```python
from build123d import *

# Parameters (mm, degrees)
F0_W     = 304.8
F0_H     = 381
F1_DEPTH = 482.6
F2_R     = 25.4
F3_R     = 12.7
F4_DEPTH = 25.4


# Not quite as in the source:
# - the program builds the solid bodies; features that only make, move or delete a surface that nothing else refers to are left out


with BuildPart() as f1:
    # F0 (on Top) → F1 (new body)
    with BuildSketch(Plane.XY):
        Rectangle(F0_W, F0_H)
    extrude(amount=F1_DEPTH)

    # F2
    f2_edges = [f1.edges().sort_by_distance(p)[0] for p in [
        (-152.4, 0, 482.6),
        (152.4, 0, 482.6),
    ]]
    fillet(f2_edges, radius=F2_R)

    # F3
    f3_edges = [f1.edges().sort_by_distance(p)[0] for p in [
        (-152.4, -190.5, 228.6),
        (-144.960512, -190.5, 475.160512),
        (0, -190.5, 482.6),
        (144.960512, -190.5, 475.160512),
        (152.4, -190.5, 228.6),
    ]]
    fillet(f3_edges, radius=F3_R)

    # F4 (cut): a face of the model
    f4_faces = [f1.faces().sort_by_distance(p)[0] for p in [
        (0, -190.5, 234.8275474118),
    ]]
    extrude(f4_faces, amount=-F4_DEPTH, mode=Mode.SUBTRACT)


solid = f1.part
```
Model file for the job. Use its own axes, mm. A direction names the side the tool comes from. Round coordinates to 2 decimals unless told otherwise and drop trailing zeros. Write each loop counter-clockwise with the first axis right and the second up, starting at its lowest first coordinate (ties: lowest second). Pieces come first, ordered by that corner, then holes. Notation, with made-up numbers: M 72.5,-27 L 76.5,-27 A17 cw 76.5,1 Z; hole C 74,-26 d10. An arc over 180 degrees is marked long. Put each result on its own line as item: value.
Item 1: Flat gauge pins, fed straight in: P1, Ø10, axis at x = 60.5, z = 102.5, coming from the -Y side; P2, Ø12.5, axis at x = -6.5, y = -181.5, coming from the -Z side. Where does each tip first touch, or does it go through?
Responses:
P1: y = -165.1
P2: z = 469.9
Item 2: Tool access for faces 4 (the flat face through (-2, -165.1, 232)), 5 (the cylindrical face through (1.78, -186.68, 478.98)): list every direction of +Z, -Z, +X, -X, +Y, -Y with a clear straight run to the whole face (end or side of a thin tool).
Responses:
face 4: -Z, -Y
face 5: +Z, +X, -X, -Y
Item 3: Cut at A-A (z = 239). List the corners of the cut face in (x, y).
Responses:
outline: M -152.4,-177.8 A12.7 ccw -139.7,-190.5 L -139.7,-165.1 L 139.7,-165.1 L 139.7,-190.5 A12.7 ccw 152.4,-177.8 L 152.4,190.5 L -152.4,190.5 Z
Item 4: Cut at B-B (x = 23.5). List the corners of the cut face in (y, z).
Responses:
outline: M -190.5,469.9 L -165.1,469.9 L -165.1,0 L 190.5,0 L 190.5,482.6 L -177.8,482.6 A12.7 ccw Z
Item 5: Probe L1, parallel to Y at x = 97, z = 186; L2, parallel to X at y = -174, z = 305.5; L3, parallel to Z at x = 133.5, y = -43. List the from-to ranges inside material, lowest first. Write a range as from..to.
Responses:
L1: -165.1..190.5
L2: -152.4..-139.7, 139.7..152.4
L3: 0..481.75
Item 6: Mould opens along X. For faces 1 (the cylindrical face through (145.16, 8.93, 474.96)), 2 (the cylindrical face through (135.88, -177.98, 466.28)), 3 (the flat face through (-2, 45, 0)) say: +X half, -X half, draft (parallel to the pull), parting line (faces both ways), or undercut.
Responses:
face 1: +X half
face 2: undercut
face 3: draft
